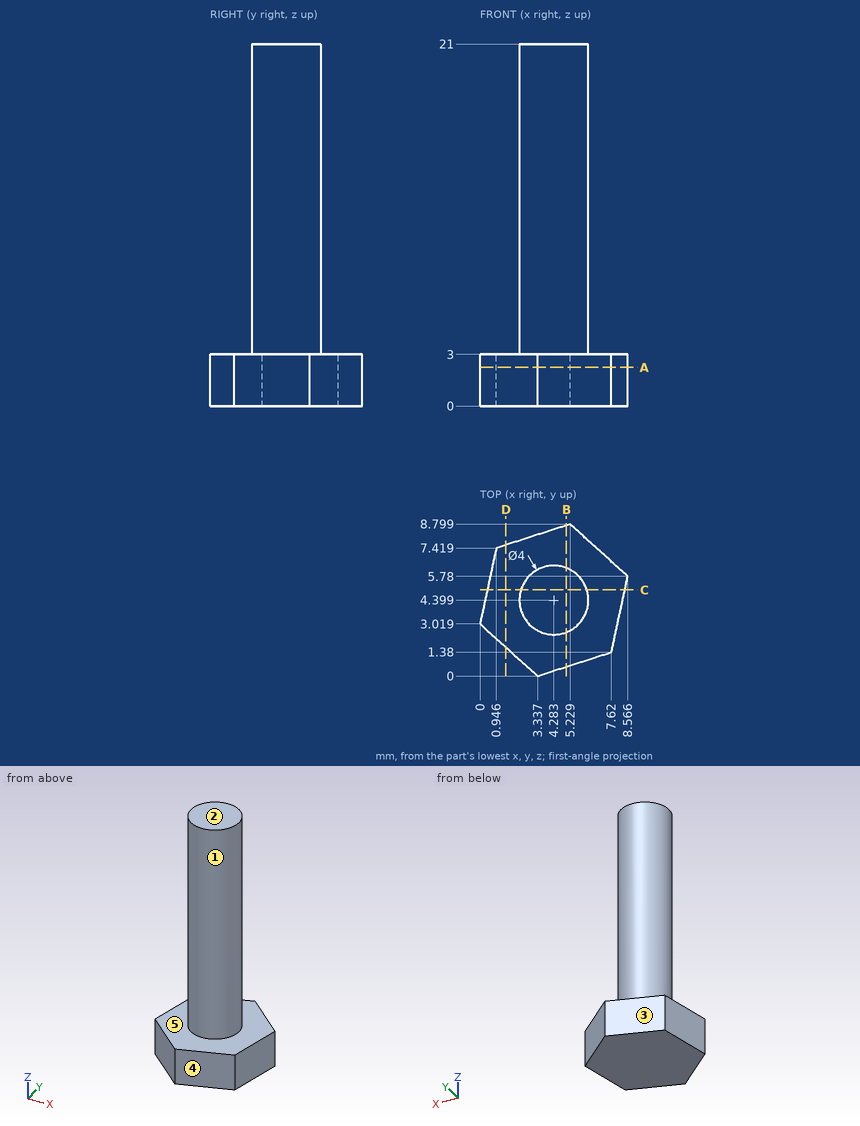
Job drawing, mm, ordinate dimensions from the low corner. One solid piece. A direction names the side the tool comes from. Round coordinates to 2 decimals unless told otherwise and drop trailing zeros. Loops run counter-clockwise (first coordinate to the right, second up) from the corner with the lowest first, then second, coordinate; pieces in that order, holes last. Notation, with made-up numbers: M -16.5,8.25 L 4.5,8.25 A23 ccw 4.5,36.25 Z; hole C -1,-38.75 d6. An arc over 180 degrees is marked long. One line per question, with ' | ' between items. Start each with the question number.
Item 1: Cut at D-D, the plane x = 1.5. Write the cut outline in (y, z), plus the area to 3 significant figures.
Item 2: Cut at B-B, the plane x = 5. Write the cut outline in (y, z) (1 decimal).
Item 3: Cut at A-A, the plane z = 2.25. Write the cut outline in (x, y), plus the area to 3 significant figures.
Item 4: Which spindle directions (+Z, -Z, +X, -X, +Y, -Y) get a long thin tool onto all of the face, cutting with end or side? Do the marked faces 4 and 5. Say none if no direction does.
Item 5: Two-plate mould, pull along Y, no slides. Class the marked faces 1, 2 and 3: pulls with the +Y half, pulls with the -Y half, needs draft (parallel to the pull), parting line crosses it, or undercut.
Item 6: Cut at C-C, the plane y = 5. Write the cut outline in (x, z) (1 decimal).
Item 7: Wall check: line 1 (Z direction, x = 7.5, y = 4.25); line 2 (X direction, y = 4.5, z = 14.5) (1 decimal); line 3 (Y direction, x = 6, z = 10.25) (1 decimal). Give the ranges that are in metal, low to high.
Item 8: Pin check, flat tips, straight feed: pin 1 Ø5 at (x, z) = (7, 13.5) entering from -Y; pin 2 Ø3 at (x, z) = (2, 6.5) entering from -Y; pin 3 Ø3 at (x, z) = (3.5, 16.5) entering from +Y. Stop position of each tip, or through.
Responses:
1) outline: M 1.66,0 L 7.6,0 L 7.6,3 L 1.66,3 Z | area: 17.8 mm²
2) outline: M 0.5,0 L 8.7,0 L 8.7,3 L 6.3,3 L 6.3,21 L 2.5,21 L 2.5,3 L 0.5,3 Z
3) outline: M 0,3.02 L 3.34,0 L 7.62,1.38 L 8.57,5.78 L 5.23,8.8 L 0.95,7.42 Z | area: 52.6 mm²
4) face 4: +Z, -Z, +X, -Y | face 5: +Z
5) face 1: parting line crosses it | face 2: needs draft | face 3: pulls with the +Y half
6) outline: M 0.4,0 L 8.4,0 L 8.4,3 L 6.2,3 L 6.2,21 L 2.4,21 L 2.4,3 L 0.4,3 Z
7) line 1: z = 0 to 3 | line 2: x = 2.3 to 6.3 | line 3: y = 3.4 to 5.4
8) pin 1: stops at y = 2.41 | pin 2: stops at y = 2.56 | pin 3: stops at y = 6.4
